Design review of the part built by this model. Coordinates are the model's own, in mm. Face numbers are marked on the shaded views. Give positions to 0.01 mm unless a question says otherwise; leave off trailing zeros. Write each loop counter-clockwise with the first axis right and the second up, starting at its lowest first coordinate (ties: lowest second). Pieces come first, ordered by that corner, then holes. Notation, with made-up numbers: (2, 20) - (42, 20) arc R18 ccw to (42, 27) - close; hole circle Ø3 at (48, -8). An arc over 180 degrees is marked (long way). Use a Markdown table: item, result. Add a question column.
```python
from build123d import *

# Parameters (mm, degrees)
F0_W     = 5
F0_H     = 5
F1_DEPTH = 50
F2_W     = 40
F2_H     = 40
F3_DEPTH = 5
F4_F1_R  = 2
F4_F2_R  = 2
F5_D     = 22
F5_DEPTH = 50
F5_START = 45
F5_TIP   = 6.6094668093


with BuildPart() as f1:
    # F0 (on Top) → F1 (new body)
    with BuildSketch(Plane.XY):
        with Locations((2.5, 2.5)):
            Rectangle(F0_W, F0_H)
    extrude(amount=F1_DEPTH)



with BuildPart() as f1b:
    # F0 (on Top) → F1, piece 2 (new body)
    with BuildSketch(Plane.XY):
        with Locations((37.5, 2.5)):
            Rectangle(F0_W, F0_H)
    extrude(amount=F1_DEPTH)


with BuildPart() as f1c:
    # F0 (on Top) → F1, piece 3 (new body)
    with BuildSketch(Plane.XY):
        with Locations((37.5, 37.5)):
            Rectangle(F0_W, F0_H)
    extrude(amount=F1_DEPTH)


with BuildPart() as f1d:
    # F0 (on Top) → F1, piece 4 (new body)
    with BuildSketch(Plane.XY):
        with Locations((2.5, 37.5)):
            Rectangle(F0_W, F0_H)
    extrude(amount=F1_DEPTH)


with BuildPart() as f1_1:
    add(f1.part)

    add(f1b.part)  # F3 merges F1b

    add(f1c.part)  # F3 merges F1c

    add(f1d.part)  # F3 merges F1d
    # F2 (on face) → F3 (join)
    with BuildSketch(Plane.XY.offset(50)):
        with Locations((20, 20)):
            Rectangle(F2_W, F2_H)
    extrude(amount=-F3_DEPTH)

    # F4: fillet of radius 2 on 20 edges, made by hand

    # F4_f1
    f4_f1_edges = [f1_1.edges().sort_by_distance(p)[0] for p in [
        (37.5, 5, 45),
        (35, 2.5, 45),
        (5, 2.5, 45),
        (2.5, 5, 45),
        (2.5, 35, 45),
        (5, 37.5, 45),
        (35, 37.5, 45),
        (37.5, 35, 45),
    ]]
    fillet(f4_f1_edges, radius=F4_F1_R)

    # F4_f2
    f4_f2_edges = [f1_1.edges().sort_by_distance(p)[0] for p in [
        (0, 20, 50),
        (20, 0, 50),
        (40, 20, 50),
        (20, 40, 50),
        (0, 0, 25),
        (40, 0, 25),
        (40, 40, 25),
        (20, 0, 45),
        (0, 20, 45),
        (20, 40, 45),
        (40, 20, 45),
        (0, 40, 25),
        (40, 5.5857864376, 44.4142135624),
        (40, 34.4142135624, 44.4142135624),
        (34.4142135624, 40, 44.4142135624),
        (5.5857864376, 40, 44.4142135624),
        (0, 34.4142135624, 44.4142135624),
        (0, 5.5857864376, 44.4142135624),
        (5.5857864376, 0, 44.4142135624),
        (34.4142135624, 0, 44.4142135624),
    ]]
    fillet(f4_f2_edges, radius=F4_F2_R)

    # F5
    # its depths count from where the whole tool has entered the part; down to there all is cleared
    with Locations(Plane(origin=(0, 0, 0), x_dir=(1, 0, 0), z_dir=(0, 0, -1)).offset(-F5_START)):
        with Locations((20, -20)):
            Hole(F5_D / 2, depth=F5_DEPTH)
            with Locations((0, 0, -(F5_DEPTH + F5_TIP / 2))):  # 118° drill point
                Cone(0, F5_D / 2, F5_TIP, mode=Mode.SUBTRACT)


solid = f1_1.part
```
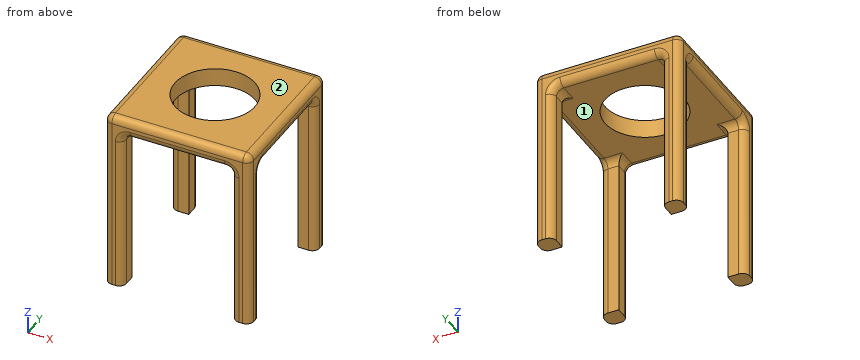
(1) Insertion check: pin 1 (1.5 mm diameter, centred on y = 34, z = 28.5, fed in from -X); pin 2 (1.5 mm diameter, centred on x = 33.5, y = 14.5, fed in from -Z); pin 3 (0.9 mm diameter, centred on y = 36, z = 26.5, fed in from +X). Each pin has a flat end and moves straight along its axis. Give the tip position at first contact, or say it passes through.
(2) For line 1 along Y through (x, z) = (20, 47.3); line 2 along X through (y, z) = (37, 20); line 3 along Z through (x, y) = (10, 27), list the stretches that pass through material, from the lowest coordinate up.
(3) Mouldability with a two-part tool opening along Y and no side actions: class the marked faces 1 and 2 as +Y half, -Y half, draft (parallel to the pull), parting line (faces both ways), or undercut.
(4) Add section C-C (z = 38). State the section outline as (x, y) points.
(5) Add section A-A (y = 20). State the section outline as (x, z) points, and give its area (3 significant figures).
Answers follow:
| question | item | result |
|---|---|---|
| 1 | pin 1 | through |
| 1 | pin 2 | z = 45 |
| 1 | pin 3 | x = 39.92 |
| 2 | line 1 | 0 to 9, 31 to 40 |
| 2 | line 2 | 0 to 5, 35 to 40 |
| 2 | line 3 | 45 to 50 |
| 3 | face 1 | undercut |
| 3 | face 2 | draft |
| 4 | outline | (0, 2) arc R2 ccw to (2, 0) - (3, 0) arc R2 ccw to (5, 2) - (5, 5) - (2, 5) arc R2 ccw to (0, 3) - close; (0, 37) arc R2 ccw to (2, 35) - (5, 35) - (5, 38) arc R2 ccw to (3, 40) - (2, 40) arc R2 ccw to (0, 38) - close; (35, 2) arc R2 ccw to (37, 0) - (38, 0) arc R2 ccw to (40, 2) - (40, 3) arc R2 ccw to (38, 5) - (35, 5) - close; (35, 35) - (38, 35) arc R2 ccw to (40, 37) - (40, 38) arc R2 ccw to (38, 40) - (37, 40) arc R2 ccw to (35, 38) - close |
| 5 | outline | (0, 47) arc R2 ccw to (2, 45) - (9, 45) - (9, 50) - (2, 50) arc R2 ccw to (0, 48) - close; (31, 45) - (38, 45) arc R2 ccw to (40, 47) - (40, 48) arc R2 ccw to (38, 50) - (31, 50) - close |
| 5 | area | 86.6 mm^2 |
